from build123d import *

# Parameters (mm, degrees)
T_SECTION_T_20_X_20_1_DEPTH = 460
SKETCH13_W                  = 20
SKETCH13_H                  = 30
CUT_EXTRUDE1_DEPTH          = 451.22216738


with BuildPart() as part:
    # Sketch12 → T section T 20 X 20(1) (new body)
    with BuildSketch(Plane.YZ):
        with BuildLine():
            Line((-10, 20), (10, 20))
            Line((10, 20), (10, 18.570314587))
            ThreePointArc((10, 18.570314587), (9.571214338, 17.520314662), (8.530000209, 17.070614622))
            Line((8.530000209, 17.070614622), (4.520436432, 16.990406743))
            ThreePointArc((4.520436432, 16.990406743), (2.459116507, 16.112327155), (1.581036919, 14.05100723))
            Line((1.581036919, 14.05100723), (1.319562646, 0.97999986))
            ThreePointArc((1.319562646, 0.97999986), (1.019762619, 0.285857108), (0.319762669, 0))
            Line((0.319762669, 0), (-0.319762669, 0))
            ThreePointArc((-0.319762669, 0), (-1.019762619, 0.285857108), (-1.319562646, 0.97999986))
            Line((-1.319562646, 0.97999986), (-1.581036919, 14.05100723))
            ThreePointArc((-1.581036919, 14.05100723), (-2.459116507, 16.112327155), (-4.520436432, 16.990406743))
            Line((-4.520436432, 16.990406743), (-8.530000209, 17.070614622))
            ThreePointArc((-8.530000209, 17.070614622), (-9.571214338, 17.520314662), (-10, 18.570314587))
            Line((-10, 18.570314587), (-10, 20))
        make_face()
    extrude(amount=T_SECTION_T_20_X_20_1_DEPTH)

    # Sketch13 → Cut-Extrude1 (cut, through all)
    with BuildSketch(Plane(origin=(10, 0, 10), x_dir=(0, -1, 0), z_dir=(-0.7071067811865464, 0, -0.7071067811865488))):
        Rectangle(SKETCH13_W, SKETCH13_H)
    extrude(amount=CUT_EXTRUDE1_DEPTH, mode=Mode.SUBTRACT)


solid = part.part
Check sheet for the modelled part. Datum: model origin and axes. Units: mm. Round coordinates to 2 decimals unless told otherwise and drop trailing zeros. Order: outer loops, then holes, each group sorted by start corner. A loop starts at its lowest first (then second) coordinate and runs counter-clockwise, first axis right, second up. Notation, with made-up numbers: M 44,-7 L 103,-7 A20 cw 103,23 Z; hole C 46.25,69 d4. An arc over 180 degrees is marked long. One line per item, written item: value. Start each with the question number.
1. Section check A-A on x = 111.5. Enter the section's corners in (y, z), and give its area (3 significant figures).
2. Section check B-B on z = 11. Enter the section's corners in (x, y).
3. Scan lines: line 1 along Z through (x, y) = (135.5, 5.25) (3 decimals); line 2 along Z through (x, y) = (319.5, -8.5); line 3 along Y through (x, z) = (406, 13.25). Record each from-to range of solid material in increasing order.
4. Gauge pin test, flat ends, axial feed: P1, Ø3, axis at x = 305.5, z = 9, coming from the +Y side; P2, Ø3, axis at y = 0, z = 4, coming from the -X side; P3, Ø4, axis at x = 394, z = 9, coming from the -Y side. Record the tip position at first contact, or that the pin passes through.
Results found:
1. outline: M -10,18.57 A1.5 ccw -8.53,17.07 L -4.52,16.99 A3 cw -1.58,14.05 L -1.32,0.98 A1 ccw -0.32,0 L 0.32,0 A1 ccw 1.32,0.98 L 1.58,14.05 A3 cw 4.52,16.99 L 8.53,17.07 A1.5 ccw 10,18.57 L 10,20 L -10,20 Z
1. area: 112 mm^2
2. outline: M 9,-1.52 L 460,-1.52 L 460,1.52 L 9,1.52 Z
3. line 1: 17.005 to 20
3. line 2: 17.07 to 20
3. line 3: -1.57 to 1.57
4. P1: y = 1.51
4. P2: x = 14.5
4. P3: y = -1.52
